For this review, take the finished solid that the model builds, in its own axes (mm). Give positions to 0.01 mm unless a question says otherwise; leave off trailing zeros. Write each loop counter-clockwise with the first axis right and the second up, starting at its lowest first coordinate (ties: lowest second). Pieces come first, ordered by that corner, then holes.
Q1. We need section A-A (y = 0.45). Write out the cut boundary in (x, z), then the cut area to 3 significant figures.
Q2. Mouldability with a two-part tool opening along Z and no side actions: class faces 1 (the flat face through (-1, 0, -1)), 2 (the cylindrical face through (-0.264, 1.288, -78.214)) as released by +Z, released by -Z, zero draft, split by the parting line, or undercut.
Q3. We need section B-B (x = 5). Write out the cut boundary in (y, z), then the cut area to 3 significant figures.
Q4. For line 1 (X direction, y = 1.55, z = 78.5); line 2 (Z direction, x = -6, y = 2.25); line 3 (Z direction, x = 1, y = 0.85), list the stretches that pass through material, from the lowest coordinate up.
```python
from build123d import *

# Parameters (mm, degrees)
SKETCH1_W           = 190.5
SKETCH1_H           = 190.5
BOSS_EXTRUDE1_DEPTH = 2.54
SKETCH2_W           = 63.5
SKETCH2_H           = 31.75
CUT_EXTRUDE1_DEPTH  = 2.54
SKETCH3_R           = 2.032
CUT_EXTRUDE2_DEPTH  = 2.54


with BuildPart() as part:
    # Sketch1 → Boss-Extrude1 (new body)
    with BuildSketch(Plane(origin=(0, 0, 0), x_dir=(1, 0, 0), z_dir=(0, 1, 0))):
        Rectangle(SKETCH1_W, SKETCH1_H)
    extrude(amount=BOSS_EXTRUDE1_DEPTH)

    # Sketch2 → Cut-Extrude1 (cut)
    with BuildSketch(Plane(origin=(0, 2.54, 0), x_dir=(1, 0, 0), z_dir=(0, 1, 0))):
        with Locations((0, -79.375)):
            Rectangle(SKETCH2_W, SKETCH2_H)
    extrude(amount=-CUT_EXTRUDE1_DEPTH, mode=Mode.SUBTRACT)

    # Sketch3 → Cut-Extrude2 (cut)
    with BuildSketch(Plane(origin=(0, 2.54, 0), x_dir=(1, 0, 0), z_dir=(0, 1, 0))):
        with Locations((0.000813673, 76.199186327)):
            Circle(SKETCH3_R)
    extrude(amount=-CUT_EXTRUDE2_DEPTH, mode=Mode.SUBTRACT)


solid = part.part
```
Computed:
1. outline: (-95.25, -95.25) - (95.25, -95.25) - (95.25, 95.25) - (31.75, 95.25) - (31.75, 63.5) - (-31.75, 63.5) - (-31.75, 95.25) - (-95.25, 95.25) - close; hole circle Ø4.06 at (0, -76.2)
1. area: 34,300 mm2
2. face 1: zero draft
2. face 2: undercut
3. outline: (0, -95.25) - (2.54, -95.25) - (2.54, 63.5) - (0, 63.5) - close
3. area: 403 mm2
4. line 1: x = -95.25 to -31.75, 31.75 to 95.25
4. line 2: z = -95.25 to 63.5
4. line 3: z = -95.25 to -77.97, -74.43 to 63.5
